The listing builds one solid part. Answer for the finished solid, in the listing's coordinates (mm). A direction names the side the tool comes from. Give positions to 0.01 mm unless a question says otherwise; leave off trailing zeros. Loops run counter-clockwise (first coordinate to the right, second up) from the corner with the lowest first, then second, coordinate; pieces in that order, holes last.
Item 1: Section C-C, the plane y = -10 is taken. Give the vertices of the cut face in (x, z).
Item 2: Section B-B, the plane z = -61 is taken. Give the vertices of the cut face in (x, y), and give its area (3 significant figures).
Item 3: Each of these flat-tipped pins is pushed along its axis until it touches: pin 1 Ø3 at (y, z) = (6.58, 60.97) entering from +X; pin 2 Ø2 at (y, z) = (2.8, 26.52) entering from -X. Where does it stop, or does it pass through?
Item 4: A tool of negligible diameter and unlimited length cuts with its end or side. For faces 4 (the face through (0.74, 12.48, -2.13)), 5 (the face through (0.74, -6, -4.68)), 6 (the face through (0.74, 3.916, -21.988)), from which of +Z, -Z, +X, -X, +Y, -Y can it reach the whole face along a straight path? Write none if from no direction.
Item 5: Section A-A, the plane x = 0.5 is taken. Give the number of separate pieces and of enclosed holes in the cut face, and give its area (3 significant figures).
Item 6: The mould has two halves that part along Z. Classify faces 1 (the face through (0.74, 1.96, -73.92)), 2 (the face through (0.74, 6.64, 62.27)), 3 (the face through (0, 3, 15)): pulls with the +Z half, pulls with the -Z half, needs draft (parallel to the pull), parting line crosses it, or undercut.
Item 7: Consider line 1 along Z through (x, y) = (0.4, -0.25); line 2 along Z through (x, y) = (0.2, 1); line 3 along Z through (x, y) = (1.25, -2). Determine where each line is inside the solid, lowest interval first.
from build123d import *

# Parameters (mm, degrees)
SKETCH_1_R      = 1.3
SKETCH_1_R_2    = 3.85
SKETCH_1_R_3    = 4
SKETCH_1_R_4    = 1.149031008
EXTRUDE_1_DEPTH = 1.5


with BuildPart() as part:
    # 草圖1 → 填料-伸長1 (new body)
    with BuildSketch(Plane(origin=(0, 0, 0), x_dir=(0, 0, -1), z_dir=(1, 0, 0))):
        with BuildLine():
            ThreePointArc((66.587683924, -5.116627236), (3.80507147, -6.050846657), (-58.633451622, -12.681082444))
            ThreePointArc((-58.633451622, -12.681082444), (-73.821962275, -1.715080477), (-61.804017134, 12.655481431))
            ThreePointArc((-61.804017134, 12.655481431), (3.033906142, 12.458288366), (67.798504291, 9.369274541))
            ThreePointArc((67.798504291, 9.369274541), (73.912446594, 1.807845069), (67.095645487, -5.12661445))
            ThreePointArc((67.095645487, -5.12661445), (66.8414518, -5.132449469), (66.587683924, -5.116627236))
        make_face()
        with Locations((-67.469663313, 0.079585479)):
            Circle(SKETCH_1_R, mode=Mode.SUBTRACT)
        with Locations((-54.469663313, 0.079585479)):
            Circle(SKETCH_1_R, mode=Mode.SUBTRACT)
        with Locations((-60.969663313, 6.579585479)):
            Circle(SKETCH_1_R, mode=Mode.SUBTRACT)
        with Locations((-60.969663313, -6.420414521)):
            Circle(SKETCH_1_R, mode=Mode.SUBTRACT)
        with Locations((66.61714054, 2.16157088)):
            Circle(SKETCH_1_R_2, mode=Mode.SUBTRACT)
        with Locations((-60.969663313, 0.079585479)):
            Circle(SKETCH_1_R_3, mode=Mode.SUBTRACT)
        with Locations((20.89210292, 3.571177524)):
            Circle(SKETCH_1_R_4, mode=Mode.SUBTRACT)
        with Locations((-26.521912025, 2.797466734)):
            Circle(SKETCH_1_R_4, mode=Mode.SUBTRACT)
    extrude(amount=EXTRUDE_1_DEPTH)


solid = part.part
Worked answers:
1. outline: (0, 39.19) - (1.5, 39.19) - (1.5, 69.27) - (0, 69.27) - close
2. outline: (0, -4.97) - (1.5, -4.97) - (1.5, 9.83) - (0, 9.83) - close
2. area: 22.2 mm2
3. pin 1: stops at x = 1.5
3. pin 2: passes through
4. face 4: +X, -X, +Y
4. face 5: +X, -X, -Y
4. face 6: +X, -X
5. separate pieces: 1
5. enclosed holes: 8
5. area: 2,650 mm2
6. face 1: pulls with the -Z half
6. face 2: undercut
6. face 3: needs draft
7. line 1: z = -73.51 to -69.62, -63.62 to 53.21, 55.73 to 56.98, 64.96 to 66.21, 68.73 to 73.92
7. line 2: z = -73.83 to -70.29, -62.95 to 53.55, 55.39 to 57.08, 64.86 to 66.55, 68.39 to 73.87
7. line 3: z = -72.62 to 57.55, 64.39 to 73.78
